```python
from build123d import *

# Parameters (mm, degrees)
BOSS_EXTRUDE1_DEPTH = 54
BOSS_EXTRUDE2_DEPTH = 18
SKETCH4_R           = 27
SKETCH4_R_2         = 15
BOSS_EXTRUDE4_DEPTH = 18
CUT_EXTRUDE1_DEPTH  = 18
BOSS_EXTRUDE5_DEPTH = 18
CUT_EXTRUDE2_DEPTH  = 9
CUT_EXTRUDE3_DEPTH  = 151.410913499


with BuildPart() as part:
    # Sketch1 → Boss-Extrude1 (new body)
    with BuildSketch(Plane(origin=(0, 0, 0), x_dir=(0, 0, -1), z_dir=(1, 0, 0))):
        Polygon((-59.11151811, 0), (73.521240549, 0), (107.462366046, 33.941125497), (94.734443984, 46.669047558), (66.065396426, 18), (-63.934603574, 18), (-81.25511165, 8), (-72.25511165, -7.588457268), align=None)
    extrude(amount=-BOSS_EXTRUDE1_DEPTH)

    # Sketch2 → Boss-Extrude2 (add)
    with BuildSketch(Plane(origin=(0, 41.184495438, 23.777879528), x_dir=(1, 0, 0), z_dir=(0, 0.8660254037844378, 0.5000000000000016))):
        Polygon((-20.230586406, -72.368990876), (-20.230586406, -122.368990876), (-11.626654027, -122.368990876), (0, -66.368990876), (-54, -66.368990876), (-45.626654027, -122.368990876), (-36.230586406, -122.368990876), (-36.230586406, -72.368990876), align=None)
    extrude(amount=-BOSS_EXTRUDE2_DEPTH)

    # Sketch4 → Boss-Extrude4 (add)
    with BuildSketch(Plane(origin=(0, -24.032698213, -24.032698213), x_dir=(1, 0, 0), z_dir=(0, 0.7071067811865462, 0.7071067811865489))):
        with Locations((-27, 99.987367753)):
            Circle(SKETCH4_R)
        with Locations((-27, 99.987367753)):
            Circle(SKETCH4_R_2, mode=Mode.SUBTRACT)
    extrude(amount=-BOSS_EXTRUDE4_DEPTH)

    # Sketch4_4 → Cut-Extrude1 (cut)
    with BuildSketch(Plane(origin=(0, -24.032698213, -24.032698213), x_dir=(1, 0, 0), z_dir=(0, 0.7071067811865462, 0.7071067811865489))):
        with BuildLine():
            Line((-37, 99.987367753), (-17, 99.987367753))
            ThreePointArc((-17, 99.987367753), (-27, 109.987367753), (-37, 99.987367753))
        make_face()
        with BuildLine():
            ThreePointArc((-37, 99.987367753), (-27, 89.987367753), (-17, 99.987367753))
            Line((-17, 99.987367753), (-37, 99.987367753))
        make_face()
    extrude(amount=-CUT_EXTRUDE1_DEPTH, mode=Mode.SUBTRACT)

    # Sketch4_5 → Boss-Extrude5 (add)
    with BuildSketch(Plane(origin=(0, -24.032698213, -24.032698213), x_dir=(1, 0, 0), z_dir=(0, 0.7071067811865462, 0.7071067811865489))):
        with BuildLine():
            Line((-17, 99.987367753), (-12, 99.987367753))
            ThreePointArc((-12, 99.987367753), (-27, 114.987367753), (-42, 99.987367753))
            Line((-42, 99.987367753), (-37, 99.987367753))
            ThreePointArc((-37, 99.987367753), (-27, 109.987367753), (-17, 99.987367753))
        make_face()
        with BuildLine():
            ThreePointArc((-42, 99.987367753), (-27, 84.987367753), (-12, 99.987367753))
            Line((-12, 99.987367753), (-17, 99.987367753))
            ThreePointArc((-17, 99.987367753), (-27, 89.987367753), (-37, 99.987367753))
            Line((-37, 99.987367753), (-42, 99.987367753))
        make_face()
    extrude(amount=-BOSS_EXTRUDE5_DEPTH)

    # Sketch4_6 → Cut-Extrude2 (cut)
    with BuildSketch(Plane(origin=(0, -24.032698213, -24.032698213), x_dir=(1, 0, 0), z_dir=(0, 0.7071067811865462, 0.7071067811865489))):
        with BuildLine():
            Line((-17, 99.987367753), (-12, 99.987367753))
            ThreePointArc((-12, 99.987367753), (-27, 114.987367753), (-42, 99.987367753))
            Line((-42, 99.987367753), (-37, 99.987367753))
            ThreePointArc((-37, 99.987367753), (-27, 109.987367753), (-17, 99.987367753))
        make_face()
        with BuildLine():
            ThreePointArc((-42, 99.987367753), (-27, 84.987367753), (-12, 99.987367753))
            Line((-12, 99.987367753), (-17, 99.987367753))
            ThreePointArc((-17, 99.987367753), (-27, 89.987367753), (-37, 99.987367753))
            Line((-37, 99.987367753), (-42, 99.987367753))
        make_face()
    extrude(amount=-CUT_EXTRUDE2_DEPTH, mode=Mode.SUBTRACT)

    # Sketch5 → Cut-Extrude3 (cut, through all)
    with BuildSketch(Plane(origin=(0, 18, 0), x_dir=(1, 0, 0), z_dir=(0, 1, 0))):
        with BuildLine():
            Line((-37.365679465, -25.934603574), (-37.365679465, 34.065396426))
            ThreePointArc((-37.365679465, 34.065396426), (-27, 44.431075891), (-16.634320535, 34.065396426))
            Line((-16.634320535, 34.065396426), (-16.634320535, -25.934603574))
            ThreePointArc((-16.634320535, -25.934603574), (-27, -36.300283039), (-37.365679465, -25.934603574))
        make_face()
    extrude(amount=-CUT_EXTRUDE3_DEPTH, mode=Mode.SUBTRACT)


solid = part.part
```
Here's how the part is built. I have some questions about the finished solid (model axes, mm). A direction names the side the tool comes from. Round coordinates to 2 decimals unless told otherwise and drop trailing zeros. Order: outer loops, then holes, each group sorted by start corner. A loop starts at its lowest first (then second) coordinate and runs counter-clockwise, first axis right, second up. Notation, with made-up numbers: M 58,19 L 84,19 A15 ccw 84,46 Z; hole C 0.25,-33.5 d5. An arc over 180 degrees is marked long. One line per question, with ' | ' between items.
1) I want a section at A-A, the plane z = -15. Write out the boundary of the cut face in (x, y), then the cut area to 3 significant figures.
Working result:
outline: M -54,0 L -37.37,0 L -37.37,18 L -54,18 Z; M -16.63,0 L 0,0 L 0,18 L -16.63,18 Z | area: 599 mm²
2) For faces 4 (the face through (-23.877, 33.383, -94.176)), 5 (the face through (-37.366, 9, -4)), 6 (the face through (-39, 0, -6)), which set-ups out of +Z, -Z, +X, -X, +Y, -Y let a thin tool reach every point of the face, with its end or its side?
Working result:
face 4: none | face 5: +Y, -Y | face 6: -Z, +X, -X, -Y
3) I want a section at C-C, the plane z = 89.5. Write out the boundary of the cut face in (x, y).
Working result:
outline: M -52.58,3.24 L -51.02,-17.54 L -36.23,-17.54 L -36.23,3.24 Z; M -20.23,-17.54 L -4.13,-17.54 L -1.98,3.24 L -20.23,3.24 Z
4) I want a section at D-D, the plane x = -3.5. Write out the boundary of the cut face in (y, z).
Working result:
outline: M -16.02,86.85 L 0,59.11 L 0,-73.52 L 43.34,-116.86 L 56.07,-104.14 L 18,-66.07 L 18,63.93 L -0.43,95.85 Z
5) For pin 1 Ø6 at (x, y) = (-36, 19) entering from +Z; pin 2 Ø5 at (x, y) = (-10.5, 8.5) entering from -Z; pin 3 Ø16 at (x, z) = (-38, -31) entering from +Y, each with a flat end and sliding along its axis, tell me the tip position at first contact or that it passes through.
Working result:
pin 1: z = 67.4 | pin 2: z = -84.52 | pin 3: y = 18
6) If we mould it in two halves opening along X, with no side actions, what happens to faces 1 (the face through (-5.895, -13.881, 101.406)), 2 (the face through (-25.047, 33.015, -87.356)), 3 (the face through (-39, 18, -2))? For each: +X half, -X half, draft (parallel to the pull), parting line (faces both ways), or undercut.
Working result:
face 1: +X half | face 2: undercut | face 3: draft
7) I want a section at B-B, the plane x = -27. Write out the boundary of the cut face in (y, z) (3 decimals).
Working result:
outline: M -10.588,77.451 L 0,59.112 L 0,36.3 L 18,36.3 L 18,63.935 L 5,86.451 Z; M 0,-73.521 L 26.87,-100.391 L 33.234,-94.027 L 29.698,-90.492 L 36.062,-84.128 L 18,-66.065 L 18,-44.431 L 0,-44.431 Z; M 41.012,-114.533 L 53.033,-126.554 L 65.761,-113.826 L 57.276,-105.341 L 50.912,-111.705 L 47.376,-108.169 Z
8) I need wall thicknesses on line 1 along X through (y, z) = (7, 9.5); line 2 along Y through (x, z) = (-4, 30); line 3 along Z through (x, y) = (-34, 6). Which ranges of each line are inside material? Lowest first, please.
Working result:
line 1: -54 to -37.37, -16.63 to 0 | line 2: 0 to 18 | line 3: -79.52 to -41.71, 33.58 to 84.72
